from build123d import *

# Parameters (mm, degrees)
F0_W        = 15.12
F0_H        = 17.76
F0_R        = 1.75
F0_W_2      = 3
F0_H_2      = 15.76
F0_W_3      = 35
F0_H_3      = 2
F1_DEPTH    = 3
F2_DEPTH    = 30.75
F4_DEPTH    = 3
F5_T4_DEPTH = 161.4443452539


# Not quite as in the source:
# - a fillet or chamfer that OpenCascade refuses, or shapes differently, is made with other operations: its cross-section is extruded or revolved along the edge and cut away or added


with BuildPart() as f1:
    # F0 (on Front) → F1 (new body)
    with BuildSketch(Plane.XZ):
        Rectangle(F0_W, F0_H)
        with Locations((-3.9189920692, -4.63)):
            Circle(F0_R, mode=Mode.SUBTRACT)
        with Locations((4.1910079308, -4.63)):
            Circle(F0_R, mode=Mode.SUBTRACT)
        Polygon((-7.56, -8.88), (-7.56, 8.88), (-44.56, 8.88), (-44.56, -6.88), (-9.56, -6.88), (-9.56, -8.88), align=None)
        with Locations((-46.06, 1)):
            Rectangle(F0_W_2, F0_H_2)
        with Locations((-27.06, -7.88)):
            Rectangle(F0_W_3, F0_H_3)
        with Locations((-46.06, -7.88)):
            Rectangle(F0_W_2, F0_H_3)
    extrude(amount=F1_DEPTH)

    # F0 (on Front) → F2 (join)
    with BuildSketch(Plane.XZ):
        with Locations((-46.06, 1)):
            Rectangle(F0_W_2, F0_H_2)
        with Locations((-46.06, -7.88)):
            Rectangle(F0_W_2, F0_H_3)
        with Locations((-27.06, -7.88)):
            Rectangle(F0_W_3, F0_H_3)
    extrude(amount=-F2_DEPTH)

    # F3 (on face) → F4 (join)
    with BuildSketch(Plane(origin=(-47.56, 0, 0), x_dir=(0, -1, 0), z_dir=(-1, 0, 0))):
        with BuildLine():
            Line((-30.75, 36.9310820997), (-30.75, 34.42))
            Line((-30.75, 34.42), (-23.2759684913, 34.42))
            Line((-23.2759684913, 34.42), (-20.25, 34.42))
            Line((-20.25, 34.42), (-20.25, 36.9310820997))
            ThreePointArc((-20.25, 36.9310820997), (-21.7144660941, 40.4666160056), (-25.25, 41.9310820997))
            Line((-25.25, 41.9310820997), (-25.75, 41.9310820997))
            ThreePointArc((-25.75, 41.9310820997), (-29.2855339059, 40.4666160056), (-30.75, 36.9310820997))
        make_face()
        with BuildLine():
            Line((-23.2759684913, 36.3402245806), (-23.2759684913, 34.42))
            Line((-23.2759684913, 34.42), (-23.922206416, 35.0770037331))
            ThreePointArc((-23.922206416, 35.0770037331), (-27.6352195224, 37.3905449889), (-23.2759684913, 37.0219396188))
            ThreePointArc((-23.2759684913, 37.0219396188), (-23.2565015161, 36.852004751), (-23.25, 36.6810820997))
            ThreePointArc((-23.25, 36.6810820997), (-23.2565015161, 36.5101594484), (-23.2759684913, 36.3402245806))
        make_face(mode=Mode.SUBTRACT)
        Polygon((-30.75, 34.42), (-30.75, 8.88), (-20.25, 8.88), (-20.25, 31.3436212872), (-23.2759684913, 34.42), align=None)
        Polygon((-23.2759684913, 34.42), (-20.25, 31.3436212872), (-20.25, 34.42), align=None)
        with BuildLine():
            Line((3, 1.0805530297), (3, -8.88))
            Line((3, -8.88), (19.3145081394, -8.88))
            Line((19.3145081394, -8.88), (16.2589368567, -5.7735253369))
            ThreePointArc((16.2589368567, -5.7735253369), (13.0770649061, -5.7472405543), (13.1033496887, -2.5653686037))
            Line((13.1033496887, -2.5653686037), (9.517170933, 1.0805530297))
            Line((9.517170933, 1.0805530297), (3, 1.0805530297))
        make_face()
        with BuildLine():
            Line((16.2589368567, -5.7735253369), (19.3145081394, -8.88))
            Line((19.3145081394, -8.88), (19.9311432727, -8.88))
            Line((19.9311432727, -8.88), (19.9311432727, -3.9194469703))
            ThreePointArc((19.9311432727, -3.9194469703), (18.4666771787, -0.3839130644), (14.9311432727, 1.0805530297))
            Line((14.9311432727, 1.0805530297), (9.517170933, 1.0805530297))
            Line((9.517170933, 1.0805530297), (13.1033496887, -2.5653686037))
            ThreePointArc((13.1033496887, -2.5653686037), (15.5507594053, -2.0942920889), (16.9311432727, -4.1694469703))
            ThreePointArc((16.9311432727, -4.1694469703), (16.7562981542, -5.0390631029), (16.2589368567, -5.7735253369))
        make_face()
        with BuildLine():
            Line((-23.922206416, 35.0770037331), (-23.2759684913, 34.42))
            Line((-23.2759684913, 34.42), (-23.2759684913, 36.3402245806))
            ThreePointArc((-23.2759684913, 36.3402245806), (-23.4969023398, 35.6563383445), (-23.922206416, 35.0770037331))
        make_face()
    extrude(amount=-F4_DEPTH)

    # F5: chamfer of 31 on 1 edges, made by hand


with BuildPart() as f5_tool2:
    # F5_s3 → F5_t4 (new body)
    with BuildSketch(Plane.XY.offset(-88.6021726269)):
        Polygon((-9.56, -0.25), (-40.56, 30.75), (-9.56, 30.75), align=None)
    extrude(amount=F5_T4_DEPTH)

    split(bisect_by=Plane.XZ, keep=Keep.BOTTOM)


with BuildPart() as f1_1:
    add(f1.part)

    # F5_t1: cut F5_tool2
    add(f5_tool2.part, mode=Mode.SUBTRACT)


solid = f1_1.part
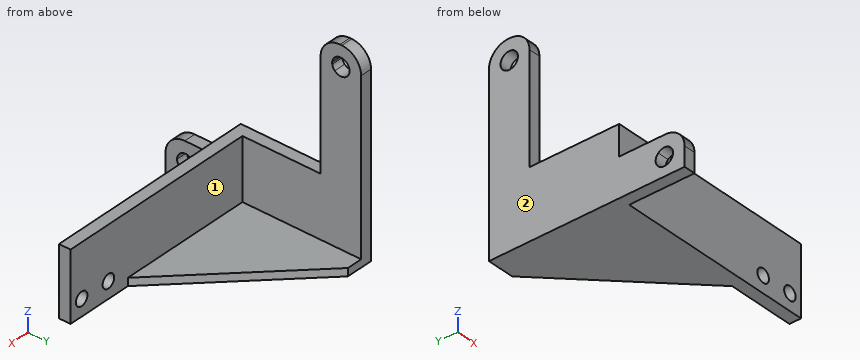
The model under review builds one solid part; all positions refer to its coordinate system, in mm. Face numbers are marked on the shaded views. A direction names the side the tool comes from. Round coordinates to 2 decimals unless told otherwise and drop trailing zeros. Loops run counter-clockwise (first coordinate to the right, second up) from the corner with the lowest first, then second, coordinate; pieces in that order, holes last. Notation, with made-up numbers: (-18, -19) - (15, -19) arc R25 cw to (15, 5) - close; hole circle Ø8 at (-13, 46.25). An arc over 180 degrees is marked (long way). Use CSV: the item, a comma, the result in double quotes.
(1) Take a section at C-C, the plane z = 3.5. Give the boundary of the cut face in (x, y), plus the area to 3 significant figures.
Working result:
outline,"(-47.56, -3) - (7.56, -3) - (7.56, 0) - (-44.56, 0) - (-44.56, 30.75) - (-47.56, 30.75) - close"
area,"258 mm^2"
(2) Take a section at B-B, the plane y = 27. Give the boundary of the cut face in (x, z), plus the area to 3 significant figures.
Working result:
outline,"(-47.56, -8.88) - (-36.81, -8.88) - (-36.81, -6.88) - (-44.56, -6.88) - (-44.56, 35) - (-47.56, 35) - close; (-47.56, 38.36) - (-44.56, 38.36) - (-44.56, 41.77) - (-47.56, 41.77) - close"
area,"157 mm^2"
(3) Clearance check with flat-ended pins moving along their axes: P1, Ø8, axis at x = -27.5, y = 3, coming from the +Z side; P2, Ø5, axis at x = -19, z = 10.5, coming from the +Y side; P3, Ø0.9, axis at x = -46, z = 16, coming from the -Y side. State where each tip first meets the part, or that it passes through.
Working result:
P1,"stops at z = 8.88"
P2,"stops at y = 0"
P3,"stops at y = 20.25"
(4) Take a section at A-A, the plane x = -22.5. Give the boundary of the cut face in (y, z).
Working result:
outline,"(-3, -8.88) - (12.69, -8.88) - (12.69, -6.88) - (0, -6.88) - (0, 8.88) - (-3, 8.88) - close"
(5) For line 1 (Z direction, x = -45.4, y = 25.5); line 2 (X direction, y = 4, z = 8.5); line 3 (Z direction, x = -20, y = -1), list the stretches that pass through material, from the lowest coordinate up.
Working result:
line 1,"z = -8.88 to 34.43, 38.93 to 41.93"
line 2,"x = -47.56 to -44.56"
line 3,"z = -8.88 to 8.88"
(6) Machinability: for the marked faces 1 and 2, which of the approach directions +Z, -Z, +X, -X, +Y, -Y give a long, thin tool a straight path to every point of the face, cutting with its end or side? Answer none if there is none.
Working result:
face 1,"+Z, +X, +Y"
face 2,"+Z, -Z, -X, +Y, -Y"
(7) Take a section at D-D, the plane z = 32. Give the boundary of the cut face in (x, y).
Working result:
outline,"(-47.56, 20.25) - (-44.56, 20.25) - (-44.56, 30.75) - (-47.56, 30.75) - close"
